Check sheet for the drawn part. Datum: minimum x, y, z corner. Units: mm. Round coordinates to 2 decimals unless told otherwise and drop trailing zeros. Write each loop counter-clockwise with the first axis right and the second up, starting at its lowest first coordinate (ties: lowest second). Pieces come first, ordered by that corner, then holes. Notation, with made-up numbers: M 55,-10.5 L 62,-10.5 A22 ccw 62,25.5 Z; hole C 66.5,52 d8. An arc over 180 degrees is marked long. Use a Markdown table: item, result.
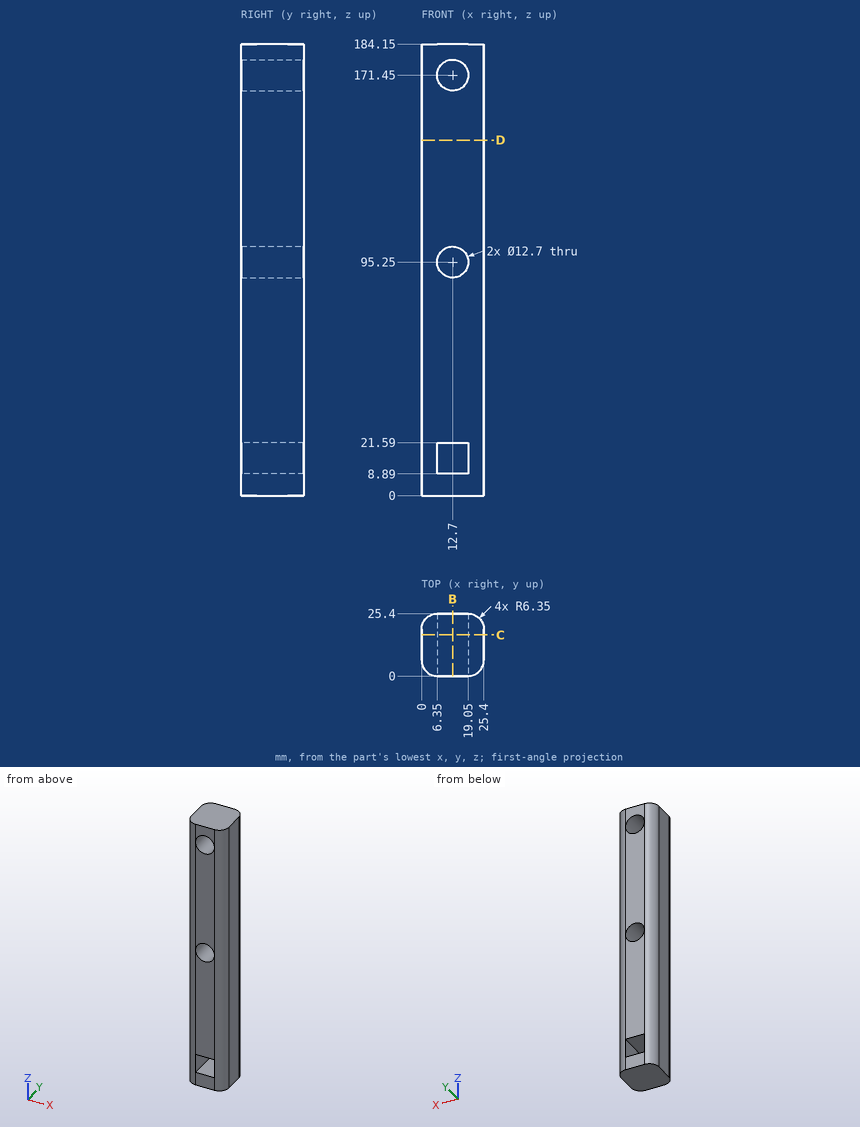
Item 1: Cross-section at B-B, the plane x = 12.7. Record the cut outline in (y, z), and give its area (3 significant figures).
Outcome:
| item | result |
|---|---|
| outline | M 0,0 L 25.4,0 L 25.4,8.89 L 0,8.89 Z; M 0,21.59 L 25.4,21.59 L 25.4,88.9 L 0,88.9 Z; M 0,101.6 L 25.4,101.6 L 25.4,165.1 L 0,165.1 Z; M 0,177.8 L 25.4,177.8 L 25.4,184.15 L 0,184.15 Z |
| area | 3,710 mm2 |
Item 2: Cross-section at C-C, the plane y = 16.75. Record the cut outline in (x, z), and give its area (3 significant figures).
Outcome:
| item | result |
|---|---|
| outline | M 0,0 L 25.4,0 L 25.4,184.15 L 0,184.15 Z; hole M 6.35,8.89 L 19.05,8.89 L 19.05,21.59 L 6.35,21.59 Z; hole C 12.7,95.25 d12.7; hole C 12.7,171.45 d12.7 |
| area | 4,260 mm2 |
Item 3: Go/stop test with flat-tipped pins: pin 1 (2 mm diameter, centred on x = 22.5, z = 46.5, fed in from +Y); pin 2 (4 mm diameter, centred on y = 15, z = 16, fed in from -X); pin 3 (1.5 mm diameter, centred on x = 5, z = 94, fed in from -Y). Record where each tip stops, or that it passes through.
Outcome:
| item | result |
|---|---|
| pin 1 | stops at y = 24.91 |
| pin 2 | stops at x = 0 |
| pin 3 | stops at y = 0.03 |
Item 4: Cross-section at D-D, the plane z = 145. Record the cut outline in (x, y).
Outcome:
| item | result |
|---|---|
| outline | M 0,6.35 A6.35 ccw 6.35,0 L 19.05,0 A6.35 ccw 25.4,6.35 L 25.4,19.05 A6.35 ccw 19.05,25.4 L 6.35,25.4 A6.35 ccw 0,19.05 Z |
Item 5: Material ranges on line 1 along Z through (x, y) = (12.7, 5); line 2 along Z through (x, y) = (14.5, 17.5); line 3 along X through (y, z) = (20.75, 93), recorded low to high. Write a range as from..to.
Outcome:
| item | result |
|---|---|
| line 1 | z = 0..8.89, 21.59..88.9, 101.6..165.1, 177.8..184.15 |
| line 2 | z = 0..8.89, 21.59..89.16, 101.34..165.36, 177.54..184.15 |
| line 3 | x = 0.23..6.76, 18.64..25.17 |
